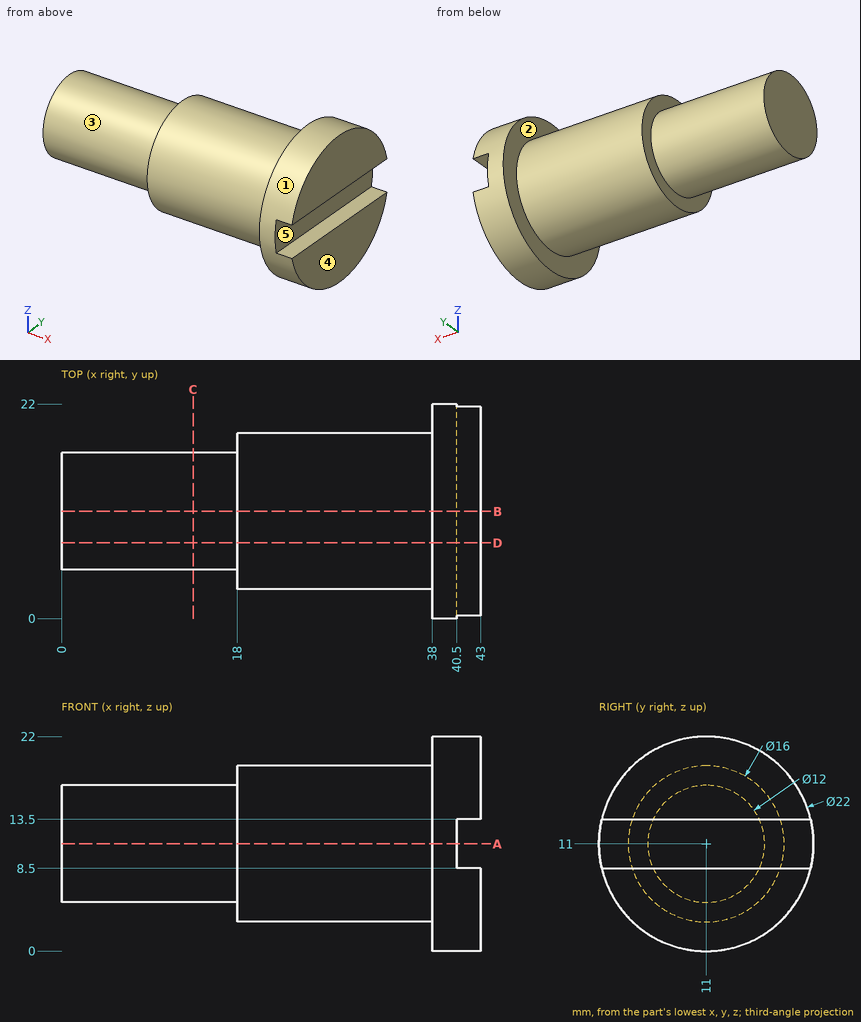
The drawing under review shows one solid part. Ordinate dimensions are in mm from its lowest x, y, z. A direction names the side the tool comes from. Give positions to 0.01 mm unless a question says otherwise; leave off trailing zeros. Write each loop counter-clockwise with the first axis right and the second up, starting at its lowest first coordinate (ties: lowest second). Pieces come first, ordered by that corner, then holes.
1. Add section C-C, the plane x = 13.5. Write out the cut boundary in (y, z).
2. Tool access review of the marked faces 1 and 2: name each direction out of +Z, -Z, +X, -X, +Y, -Y from which nothing blocks a thin tool from reaching the whole face with its end or side.
3. Wall thickness on L1, parallel to X at y = 19.75, z = 10; L2, parallel to X at y = 4.25, z = 9.5; L3, parallel to Y at x = 21.5, z = 11: over which ranges is each line inside the solid? List them lowest first.
4. Add section D-D, the plane y = 7.75. Write out the cut boundary in (x, z), plus the area to 3 significant figures.
5. Draft analysis for pull direction Z (two halves, no side actions). For the marked faces 3, 4 and 5, state which applies: +Z half, -Z half, draft (parallel to the pull), parting line (faces both ways), or undercut.
6. Add section A-A, the plane z = 11. Write out the cut boundary in (x, y).
7. For P1, Ø5, axis at x = 23.5, y = 7.5, coming from the -Z side; P2, Ø12, axis at x = 10, z = 4, coming from the -Y side; P3, Ø4, axis at x = 8, y = 11.5, coming from the -Z side, all flat-tipped, find the tip position at first contact; note any pin that passes through.
8. Add section B-B, the plane y = 11. Write out the cut boundary in (x, z), plus the area to 4 significant figures.
Worked answers:
1. outline: circle Ø12 at (11, 11)
2. face 1: +X, -X
2. face 2: -X
3. L1: x = 38 to 40.5
3. L2: x = 18 to 40.5
3. L3: y = 3 to 19
4. outline: (0, 5.96) - (18, 5.96) - (18, 3.69) - (38, 3.69) - (38, 0.49) - (43, 0.49) - (43, 8.5) - (40.5, 8.5) - (40.5, 13.5) - (43, 13.5) - (43, 21.51) - (38, 21.51) - (38, 18.31) - (18, 18.31) - (18, 16.04) - (0, 16.04) - close
4. area: 567 mm2
5. face 3: parting line
5. face 4: draft
5. face 5: undercut
6. outline: (0, 5) - (18, 5) - (18, 3) - (38, 3) - (38, 0) - (40.5, 0) - (40.5, 22) - (38, 22) - (38, 19) - (18, 19) - (18, 17) - (0, 17) - close
7. P1: stops at z = 3.06
7. P2: stops at y = 5.08
7. P3: stops at z = 5
8. outline: (0, 5) - (18, 5) - (18, 3) - (38, 3) - (38, 0) - (43, 0) - (43, 8.5) - (40.5, 8.5) - (40.5, 13.5) - (43, 13.5) - (43, 22) - (38, 22) - (38, 19) - (18, 19) - (18, 17) - (0, 17) - close
8. area: 633.5 mm2
